Source: CAD feature listing. Evaluate the final solid. Frame: model axes, mm. Give positions to 0.01 mm unless a question says otherwise; leave off trailing zeros. Write each loop counter-clockwise with the first axis right and the second up, starting at its lowest first coordinate (ties: lowest second). Pieces come first, ordered by that corner, then holes. Notation, with made-up numbers: (20.25, 67) -> (57.25, 67) arc R11 cw to (57.25, 81) -> close; hole circle Ø10 at (47.25, -20.75). An arc over 180 degrees is marked (long way). Answer as a JSON object with one key per item and string values. Group by question number.
Item 1: Section query C-C on z = -38. Return the cut outline in (x, y), plus the area to 3 significant figures.
Item 2: Section query A-A on y = 0. Return the cut outline in (x, z), plus the area to 3 significant figures.
Item 3: Ray query, probe 1 along Z at (x, y) = (14.5, 17.5); probe 2 along X at (y, z) = (11, -106.5); probe 3 along X at (y, z) = (-15, 77). Return the intervals inside material, ascending. Write a range as from..to.
Item 4: First-contact query: pin 1 Ø2 at (x, y) = (-14, 4) entering from +Z; pin 2 Ø6 at (x, y) = (7, 13) entering from -Z. Flat tips, straight axial feed; report the tip coordinate or a pass-through.
from build123d import *

# Parameters (mm, degrees)
SKETCH_1_R      = 6
EXTRUDE_1_DEPTH = 230
SKETCH_2_W      = 40
SKETCH_2_H      = 40
EXTRUDE_2_DEPTH = 225
FILLET_1_R      = 10


with BuildPart() as part:
    # 草图1 → 凸台-拉伸1 (new, symmetric)
    with BuildSketch(Plane.XY):
        Circle(SKETCH_1_R)
    extrude(amount=EXTRUDE_1_DEPTH, both=True)

    # 草图2 → 凸台-拉伸2 (add, symmetric)
    with BuildSketch(Plane.XY):
        Rectangle(SKETCH_2_W, SKETCH_2_H)
    extrude(amount=EXTRUDE_2_DEPTH, both=True)

    # 圆角1
    fillet_1_edges = [part.edges().sort_by_distance(p)[0] for p in [
        (20, -20, 0),
        (20, 20, 0),
        (-20, 20, 0),
        (-20, -20, 0),
    ]]
    fillet(fillet_1_edges, radius=FILLET_1_R)


solid = part.part
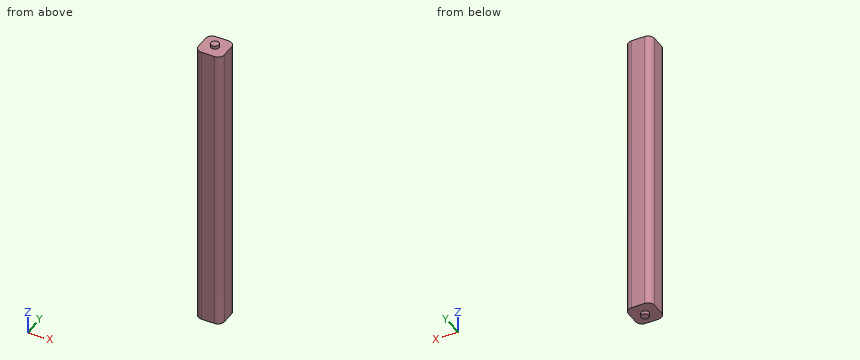
Worked answers:
{
 "1": {"outline": "(-20, -10) arc R10 ccw to (-10, -20) -> (10, -20) arc R10 ccw to (20, -10) -> (20, 10) arc R10 ccw to (10, 20) -> (-10, 20) arc R10 ccw to (-20, 10) -> close", "area": "1,510 mm^2"},
 "2": {"outline": "(-20, -225) -> (-6, -225) -> (-6, -230) -> (6, -230) -> (6, -225) -> (20, -225) -> (20, 225) -> (6, 225) -> (6, 230) -> (-6, 230) -> (-6, 225) -> (-20, 225) -> close", "area": "18,100 mm^2"},
 "3": {"probe 1": "-225..225", "probe 2": "-19.95..19.95", "probe 3": "-18.66..18.66"},
 "4": {"pin 1": "z = 225", "pin 2": "z = -225"}
}
